Check sheet for the modelled part. Datum: model origin and axes. Units: mm. Face numbers are marked on the shaded views. A direction names the side the tool comes from. Give positions to 0.01 mm unless a question says otherwise; leave off trailing zeros. Order: outer loops, then holes, each group sorted by start corner. A loop starts at its lowest first (then second) coordinate and runs counter-clockwise, first axis right, second up.
Item 1: Release check for a two-part mould opening along X. For the marked faces 1, 2, 3 and 4 record: released by +X, released by -X, zero draft, split by the parting line, or undercut.
Item 2: Gauge pin test, flat ends, axial feed: P1, Ø20, axis at x = 9.5, z = 29, coming from the -Y side; P2, Ø9.5, axis at y = -35, z = 26.5, coming from the -X side; P3, Ø4, axis at y = 15, z = 36.5, coming from the +X side; P4, Ø8, axis at x = 8, z = 38, coming from the -Y side. Record the tip position at first contact, or that the pin passes through.
Item 3: Sectioned sample at C-C on z = 28. Record the boundary of the cut face in (x, y).
Item 4: Sectioned sample at D-D on y = -27. Record the boundary of the cut face in (x, z).
Item 5: Material ranges on line 1 along Y through (x, z) = (4, 6); line 2 along Z through (x, y) = (-6, 9); line 3 along X through (y, z) = (0, 23), recorded low to high.
Item 6: Access from +Z, -Z, +X, -X, +Y, -Y to the whole of each face (thin tool, end or side, straight path). Record for the marked faces 5, 6, 7 and 8.
Item 7: Sectioned sample at B-B on y = 0. Record the boundary of the cut face in (x, z).
Item 8: Sectioned sample at A-A on x = 4. Record the boundary of the cut face in (y, z), and give its area (3 significant figures).
Autodesk Fusion 360 part; units mm, degrees
sketch "Sketch1" plane through (0, 0, 0) normal (0, 0, 1) x (1, 0, 0)
  line L0 (12.9814, 44) -> (-40, 44)
  line L1 (-40, -44) -> (12.9814, -44)
  circle A0 centre (4, -25) radius 5
  circle A1 centre (4, 25) radius 5
  line L2 (40, -25) -> (52.3485, -14.44)
  line L3 (40, 25) -> (52.3485, 14.44)
  line L4 (40, 25) -> (21.4304, 40.88)
  line L5 (40, -25) -> (21.4304, -40.88)
  circle A2 centre (-46, 0) radius 9.5
  arc A3 (-40, -25) -> (-46, -19) centre (-46, -25) ccw
  arc A4 (52.3485, -14.44) -> (52.3485, 14.44) centre (40, 0) ccw
  arc A5 (12.9814, -44) -> (21.4304, -40.88) centre (12.9814, -31) ccw
  line L6 (-40, -25) -> (-40, -44)
  arc A6 (-46, 19) -> (-46, -19) centre (-46, 0) ccw
  line L7 (-40, 44) -> (-40, 25)
  line L8 (-40, 19) -> (-40, 18.0278)
  arc A7 (-46, 19) -> (-40, 25) centre (-46, 25) ccw
  arc A8 (21.4304, 40.88) -> (12.9814, 44) centre (12.9814, 31) ccw
  line L9 (-40, 0) -> (-36.5, 0) construction
  line L10 (0, 0) -> (4, 0) construction
  line L11 (4, 20) -> (4, 19) construction
  line L12 (20.8025, 19) -> (-35, 19) construction
  line L13 (-35, -19) -> (20, -19) construction
  line L14 (-20, -5) -> (-20, 5)
  line L15 (-24, 5) -> (-20, 5)
  line L16 (-24, -5) -> (-20, -5)
  line L17 (-24, 19) -> (-24, 5)
  line L18 (-24, -5) -> (-24, -19)
  arc A9 (-24, -19) -> (-27, -22) centre (-24, -22) ccw
  arc A10 (-27, 22) -> (-24, 19) centre (-24, 22) ccw
  line L19 (-27, 44) -> (-27, 22)
  line L20 (-27, -22) -> (-27, -44)
  line L21 (-40, 44) -> (-27, 44)
  line L22 (-40, -44) -> (-27, -44)
  line L23 (-70, 0) -> (52.6501, 0) construction
  dimension "d2" = 88
  dimension "d3" = 19
  dimension "d8" = 10
  dimension "d9" = 10
  dimension "d13" = 19
  dimension "d14" = 19
  dimension "d15" = 6
  dimension "d16" = 6
  dimension "d19" = 13
  dimension "d20" = 16
  dimension "d21" = 19
  dimension "d22" = 19
  dimension "d23" = 3
  dimension "d24" = 3
  dimension "d25" = 20
  dimension "d26" = 5
  dimension "d27" = 5
  dimension "d46" = 44
  dimension "d47" = 44
extrude "Extrude1" add sketch "Sketch1" along normal blind 10
sketch "Sketch2" plane through (0, 0, 10) normal (0, 0, 1) x (-1, 0, 0)
  circle A0 centre (-4, -25) radius 5
  circle A1 centre (-4, 25) radius 5
  circle A2 centre (46, 0) radius 9.5
  line L0 (-52.3485, -14.44) -> (-21.4304, -40.88)
  arc A3 (-21.4304, -40.88) -> (-12.9814, -44) centre (-12.9814, -31) ccw
  line L1 (-12.9814, -44) -> (40, -44)
  line L2 (40, -44) -> (40, -25)
  arc A4 (46, -19) -> (40, -25) centre (46, -25) ccw
  arc A5 (46, -19) -> (46, 19) centre (46, 0) ccw
  arc A6 (40, 25) -> (46, 19) centre (46, 25) ccw
  line L3 (40, 25) -> (40, 44)
  line L4 (40, 44) -> (-12.9814, 44)
  arc A7 (-12.9814, 44) -> (-21.4304, 40.88) centre (-12.9814, 31) ccw
  line L5 (-21.4304, 40.88) -> (-52.3485, 14.44)
  arc A8 (-52.3485, 14.44) -> (-52.3485, -14.44) centre (-40, 0) ccw
  line L6 (40, -44) -> (27, -44)
  line L7 (24, -19) -> (24, -5)
  line L8 (20, -5) -> (20, 5)
  line L9 (24, 5) -> (24, 19)
  circle A9 centre (46, 0) radius 9.5
  line L10 (40, 44) -> (27, 44)
  line L11 (40, 44) -> (40, 25)
  line L12 (40, -44) -> (40, -25)
  arc A10 (40, 25) -> (46, 19) centre (46, 25) ccw
  arc A11 (46, -19) -> (46, 19) centre (46, 0) ccw
  line L13 (40, -44) -> (40, -25) construction
  line L14 (40, 25) -> (40, 44) construction
  arc A12 (24, 19) -> (27, 22) centre (24, 22) ccw
  arc A13 (46, -19) -> (40, -25) centre (46, -25) ccw
  arc A14 (27, -22) -> (24, -19) centre (24, -22) ccw
  line L15 (24, 5) -> (20, 5)
  line L16 (24, -5) -> (20, -5)
  line L17 (27, -44) -> (27, -22) construction
  line L18 (27, 22) -> (27, 44) construction
  line L19 (27, -44) -> (27, -22)
  line L20 (27, 22) -> (27, 44)
  dimension "d28" = 13
  dimension "d35" = 3
  dimension "d36" = 3
  dimension "d37" = 19
  dimension "d39" = 6
  dimension "d40" = 6
extrude "Extrude2" add sketch "Sketch2" along normal blind 40 contours L1 L2 A4 A5 A6 L3 L4 L6 L7 L8 L9 L10 L11 L12 A10 A11 A12 A13 A14 L15 L16 L19 L20
sketch "Sketch3" plane through (0, 0, 0) normal (0, 1, 0) x (1, 0, 0)
  line L0 (-20, -50) -> (-20, -10)
  line L1 (-20, -10) -> (44, -10)
  line L2 (44, -10) -> (-20, -50)
  dimension "d43" = 64
extrude "Extrude3" add sketch "Sketch3" along normal mid plane 10
equation "d20 = 13 mm + 3 mm"
equation "d43 = 67 mm - 3 mm"
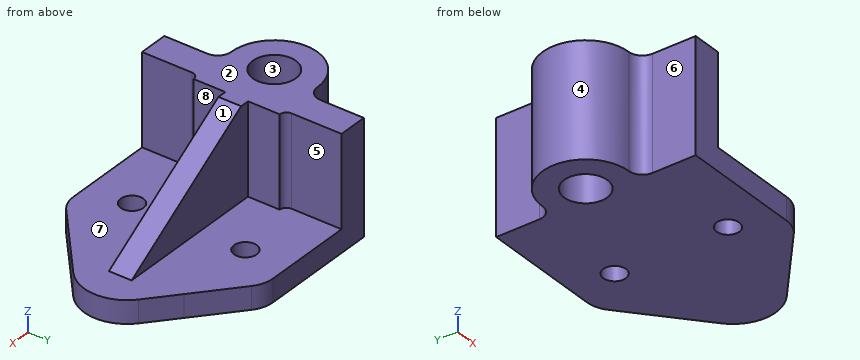
Report:
1. face 1: released by +X
1. face 2: zero draft
1. face 3: undercut
1. face 4: released by -X
2. P1: stops at y = -5
2. P2: stops at x = -40
2. P3: stops at x = -24
2. P4: passes through
3. outline: (-46, -19) arc R6 cw to (-40, -25) - (-40, -44) - (-27, -44) - (-27, -22) arc R3 cw to (-24, -19) - (-24, -5) - (15.2, -5) - (15.2, 5) - (-24, 5) - (-24, 19) arc R3 cw to (-27, 22) - (-27, 44) - (-40, 44) - (-40, 25) arc R6 cw to (-46, 19) arc R19 ccw to start; hole circle Ø19 at (-46, 0)
4. outline: (-40, 0) - (-0.58, 0) - (-0.58, 10) - (-27, 10) - (-27, 50) - (-40, 50) - close; (8.58, 0) - (37.66, 0) - (37.66, 10) - (8.58, 10) - close
5. line 1: y = -44 to -30, -20 to 20, 30 to 44
5. line 2: z = 0 to 10
5. line 3: x = -65 to -55.5, -36.5 to 23.2
6. face 5: +Z, +X, +Y
6. face 6: +Z, -Z, -X, -Y
6. face 7: +Z, +X
6. face 8: +Z, +X, -Y
7. outline: (-65, 0) - (-55.5, 0) - (-55.5, 50) - (-65, 50) - close; (-36.5, 0) - (59, 0) - (59, 10) - (44, 10) - (-20, 50) - (-36.5, 50) - close
8. outline: (-44, 0) - (-30, 0) - (-30, 10) - (-44, 10) - close; (-20, 0) - (20, 0) - (20, 10) - (5, 10) - (5, 35) - (-5, 35) - (-5, 10) - (-20, 10) - close; (30, 0) - (44, 0) - (44, 10) - (30, 10) - close
8. area: 930 mm2
